```python
from build123d import *

# Parameters (mm, degrees)
AUFSATZ_LINEAR_AUSTRAGEN1_DEPTH = 1200
SKIZZE2_R                       = 3.45
SCHNITT_LINEAR_AUSTRAGEN1_DEPTH = 30


with BuildPart() as part:
    # Skizze1 → Aufsatz-Linear austragen1 (new body)
    with BuildSketch(Plane(origin=(0, 0, 0), x_dir=(1, 0, 0), z_dir=(0, 1, 0))):
        Polygon((-4.1, -20), (-4.1, -8), (4.1, -8), (4.1, -20), (20, -20), (20, -4.1), (8, -4.1), (8, 4.1), (20, 4.1), (20, 20), (4.1, 20), (4.1, 8), (-4.1, 8), (-4.1, 20), (-20, 20), (-20, 4.1), (-8, 4.1), (-8, -4.1), (-20, -4.1), (-20, -20), align=None)
    extrude(amount=AUFSATZ_LINEAR_AUSTRAGEN1_DEPTH)

    # Skizze2 → Schnitt-Linear austragen1 (cut)
    with BuildSketch(Plane(origin=(0, 1200, 0), x_dir=(1, 0, 0), z_dir=(0, 1, 0))):
        with Locations(Location((0, 0, 0), (0, 0, 270))):
            Circle(SKIZZE2_R)
    extrude(amount=-SCHNITT_LINEAR_AUSTRAGEN1_DEPTH, mode=Mode.SUBTRACT)


solid = part.part
```
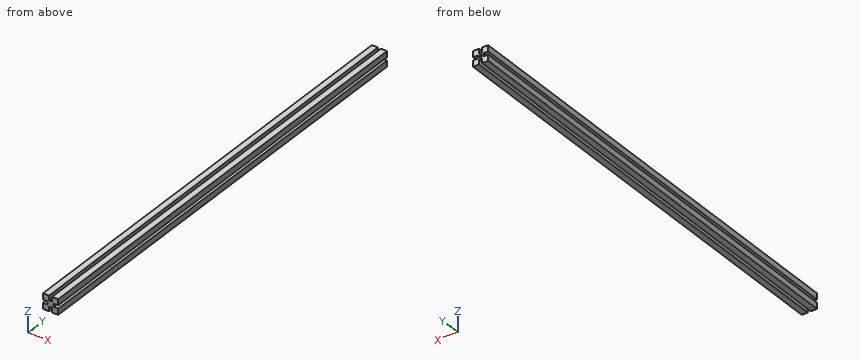
For this review, take the finished solid that the model builds, in its own axes (mm). Round coordinates to 2 decimals unless told otherwise and drop trailing zeros. Write each loop counter-clockwise with the first axis right and the second up, starting at its lowest first coordinate (ties: lowest second). Pieces come first, ordered by that corner, then holes. Notation, with made-up numbers: (47, 58) -> (55, 58) arc R22 ccw to (55, 95) -> close; hole circle Ø7 at (-16, 80.5). An arc over 180 degrees is marked (long way). One line per question, with ' | ' between items. Start each with the question number.
1) Add section A-A (y = 368). Write out the cut boundary in (x, z).
2) For pin 1 Ø4 at (x, y) = (-1, 455.5) entering from +Z; pin 2 Ø2 at (x, z) = (1, 0.5) entering from +Y; pin 3 Ø2.5 at (y, z) = (773.5, -0.5) entering from -X, all flat-tipped, find the tip position at first contact; note any pin that passes through.
3) Wall thickness on line 1 along Z through (x, y) = (13.5, 56); line 2 along X through (y, z) = (1185, 0): over which ranges is each line inside the solid? List them lowest first.
Reported:
1) outline: (-20, -20) -> (-4.1, -20) -> (-4.1, -8) -> (4.1, -8) -> (4.1, -20) -> (20, -20) -> (20, -4.1) -> (8, -4.1) -> (8, 4.1) -> (20, 4.1) -> (20, 20) -> (4.1, 20) -> (4.1, 8) -> (-4.1, 8) -> (-4.1, 20) -> (-20, 20) -> (-20, 4.1) -> (-8, 4.1) -> (-8, -4.1) -> (-20, -4.1) -> close
2) pin 1: stops at z = 8 | pin 2: stops at y = 1170 | pin 3: stops at x = -8
3) line 1: z = -20 to -4.1, 4.1 to 20 | line 2: x = -8 to -3.45, 3.45 to 8
